from build123d import *

# Parameters (mm, degrees)
SKETCH1_R           = 7
BOSS_EXTRUDE1_DEPTH = 5
FILLET1_R           = 2


with BuildPart() as part:
    # Sketch1 → Boss-Extrude1 (new body)
    with BuildSketch(Plane.XY):
        with BuildLine():
            Line((0, 0), (0, -38))
            Line((0, -38), (5.5, -38))
            Line((5.5, -38), (5.5, 0))
            ThreePointArc((5.5, 0), (2.75, 23.680646386), (0, 0))
        make_face()
        with Locations((2.75, 11.680646386)):
            Circle(SKETCH1_R, mode=Mode.SUBTRACT)
    extrude(amount=BOSS_EXTRUDE1_DEPTH)

    # Fillet1
    fillet1_edges = [part.edges().sort_by_distance(p)[0] for p in [
        (5.5, 0, 2.5),
        (5.5, -38, 2.5),
        (0, -38, 2.5),
        (0, 0, 2.5),
    ]]
    fillet(fillet1_edges, radius=FILLET1_R)


solid = part.part
Work out the finished part from the listing and answer in its coordinate system (mm). A direction names the side the tool comes from. Round coordinates to 2 decimals unless told otherwise and drop trailing zeros. Write each loop counter-clockwise with the first axis right and the second up, starting at its lowest first coordinate (ties: lowest second). Pieces come first, ordered by that corner, then holes.
1) Given pin 1 Ø10 at (x, y) = (-3.5, -5.5) entering from +Z; pin 2 Ø1.5 at (y, z) = (-25.5, 2.5) entering from -X, each flat-ended and moving along its own axis, determine where each tip first touches the part or whether it passes through.
2) A cutting plane is placed at B-B (z = 2.45). Give the vertices of the cut face in (x, y), plus the area to 3 significant figures.
3) A cutting plane is placed at D-D (x = 7.5). Give the vertices of the cut face in (y, z), plus the area to 3 significant figures.
4) Straight lines are drawn through the part: line 1 (Y direction, x = 2.75, z = 3.35); line 2 (X direction, y = -30, z = 4.05); line 3 (Y direction, x = -0.75, z = 1.3). For each, find the intervals that lie inside material, in ascending order.
5) A cutting plane is placed at A-A (x = 2.75). Give the vertices of the cut face in (y, z), plus the area to 3 significant figures.
6) The mould has two halves that part along X. Classify faces 4 (the cylindrical face through (3.22, 23.67, 2.46)), 5 (the cylindrical face through (0.57, -37.4, 2.54)), 6 (the cylindrical face through (1.84, 18.62, 2.46)): pulls with the +X half, pulls with the -X half, needs draft (parallel to the pull), parting line crosses it, or undercut.
7) A tool of negligible diameter and unlimited length cuts with its end or side. For faces 1 (the flat face through (2, -2, 5)), 2 (the flat face through (0, -19, 2)), 3 (the flat face through (5.5, -19, 2)), from which of +Z, -Z, +X, -X, +Y, -Y can it reach the whole face along a straight path? Write none if from no direction.
8) A cutting plane is placed at C-C (y = -11.5). Give the vertices of the cut face in (x, z).
Completed:
1. pin 1: stops at z = 5
1. pin 2: stops at x = 0
2. outline: (-1.32, 0.39) arc R2 cw to (0, -1.49) - (0, -36) arc R2 ccw to (2, -38) - (3.5, -38) arc R2 ccw to (5.5, -36) - (5.5, -1.49) arc R2 cw to (6.82, 0.39) arc R12 ccw (long way) to start; hole circle Ø14 at (2.75, 11.68)
2. area: 505 mm2
3. outline: (0.66, 0) - (6.54, 0) - (6.54, 5) - (0.66, 5) - close; (16.82, 0) - (22.7, 0) - (22.7, 5) - (16.82, 5) - close
3. area: 58.8 mm2
4. line 1: y = -38 to 4.68, 18.68 to 23.68
4. line 2: x = 0 to 5.5
4. line 3: y = 0.07 to 5.62, 17.74 to 23.16
5. outline: (-38, 0) - (4.68, 0) - (4.68, 5) - (-38, 5) - close; (18.68, 0) - (23.68, 0) - (23.68, 5) - (18.68, 5) - close
5. area: 238 mm2
6. face 4: parting line crosses it
6. face 5: pulls with the -X half
6. face 6: undercut
7. face 1: +Z, +X, -X, +Y, -Y
7. face 2: +Z, -Z, -X, -Y
7. face 3: +Z, -Z, +X, -Y
8. outline: (0, 0) - (5.5, 0) - (5.5, 5) - (0, 5) - close
